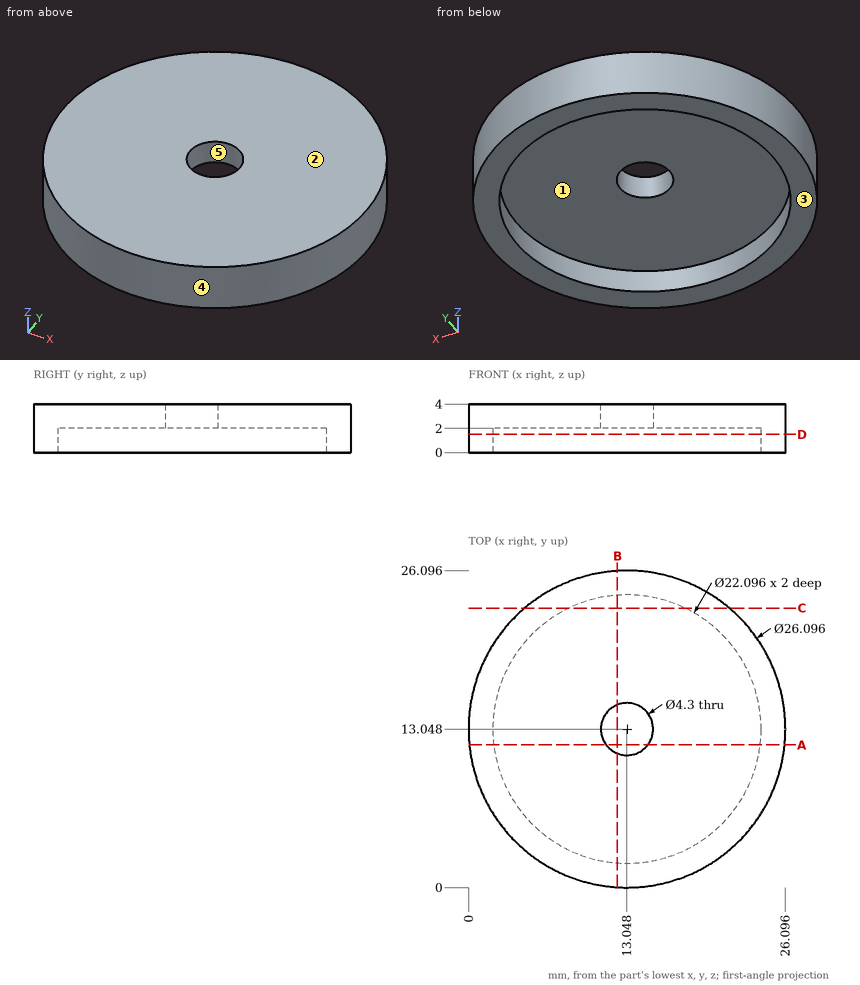
Geometry check sheet. Reference: drawing and pictorial views, mm from the part's lowest x, y, z. A direction names the side the tool comes from. Coordinates: 2 decimals unless noted, no trailing zeros. Write each loop counter-clockwise with the first axis right and the second up, starting at its lowest first coordinate (ties: lowest second). Pieces come first, ordered by that corner, then holes. Notation, with made-up numbers: (48, -12.75) - (68, -12.75) arc R23 cw to (68, 8.25) - close; hole circle Ø9 at (66, 46.5). An arc over 180 degrees is marked (long way). One line per question, with ' | ' between items. Start each with the question number.
1. Material ranges on line 1 along Z through (x, y) = (6.25, 11.5); line 2 along X through (y, z) = (13.25, 1.7) (1 decimal); line 3 along X through (y, z) = (7, 0.2) (1 decimal), recorded low to high.
2. Section check C-C (y = 23). Enter the section's corners in (x, z).
3. Access from +Z, -Z, +X, -X, +Y, -Y to the whole of each face (thin tool, end or side, straight path). Record for the marked faces 1 and 2.
4. Draft check along Y on the marked faces 3, 4 and 5. Enter one of: released by +Y, released by -Y, zero draft, split by the parting line, or undercut.
5. Section check B-B (x = 12.25). Enter the section's corners in (y, z) (1 decimal).
6. Section check A-A (y = 11.75). Enter the section's corners in (x, z) (1 decimal).
7. Section check D-D (z = 1.5). Enter the section's corners in (x, y).
8. Gauge pin test, flat ends, axial feed: P1, Ø7, axis at x = 13.05, y = 13.05, coming from the +Z side; P2, Ø6.5, axis at x = 11.5, y = 12, coming from the -Z side; P3, Ø1.5, axis at x = 21.5, z = 2.5, coming from the -Y side (1 decimal); P4, Ø1, axis at y = 11, z = 1.5, coming from the +X side. Record the tip position at first contact, or that the pin passes through.
Computed values:
1) line 1: 2 to 4 | line 2: 0 to 2, 24.1 to 26.1 | line 3: 1.5 to 3.8, 22.3 to 24.6
2) outline: (4.61, 0) - (8.25, 0) - (8.25, 2) - (17.85, 2) - (17.85, 0) - (21.49, 0) - (21.49, 4) - (4.61, 4) - close
3) face 1: -Z | face 2: +Z, +X, -X, +Y, -Y
4) face 3: zero draft | face 4: split by the parting line | face 5: undercut
5) outline: (0, 0) - (2, 0) - (2, 2) - (11.1, 2) - (11.1, 4) - (0, 4) - close; (15, 2) - (24.1, 2) - (24.1, 0) - (26.1, 0) - (26.1, 4) - (15, 4) - close
6) outline: (0.1, 0) - (2.1, 0) - (2.1, 2) - (11.3, 2) - (11.3, 4) - (0.1, 4) - close; (14.8, 2) - (24, 2) - (24, 0) - (26, 0) - (26, 4) - (14.8, 4) - close
7) outline: circle Ø26.1 at (13.05, 13.05); hole circle Ø22.1 at (13.05, 13.05)
8) P1: z = 4 | P2: z = 2 | P3: y = 2.5 | P4: x = 26
